Geometry check sheet. Reference: the model listing, model coordinates, mm. A direction names the side the tool comes from. Round coordinates to 2 decimals unless told otherwise and drop trailing zeros. Write each loop counter-clockwise with the first axis right and the second up, starting at its lowest first coordinate (ties: lowest second). Pieces come first, ordered by that corner, then holes. Notation, with made-up numbers: (61.25, 59.25) -> (74.25, 59.25) arc R13 cw to (74.25, 63.25) -> close; hole circle Ø4 at (-10.5, 35.5). An arc over 180 degrees is marked (long way). One line per question, with ' | ' between items.
```python
from build123d import *

# Parameters (mm, degrees)
SKETCH7_R           = 5
BOSS_EXTRUDE5_DEPTH = 12
SKETCH8_R           = 6
BOSS_EXTRUDE6_DEPTH = 2
SKETCH9_R           = 4.5
BOSS_EXTRUDE7_DEPTH = 10
FILLET2_R           = 20
FILLET3_R           = 10
FILLET5_R           = 3


with BuildPart() as part:
    # Sketch7 → Boss-Extrude5 (new body)
    with BuildSketch(Plane(origin=(0, 0, 0), x_dir=(1, 0, 0), z_dir=(0, 1, 0))):
        with BuildLine():
            Line((-105.5, 30), (-105.5, 0))
            ThreePointArc((-105.5, 0), (-95.5, -10), (-85.5, 0))
            Line((-85.5, 0), (-85.5, 15))
            Line((-85.5, 15), (-10, 15))
            Line((-10, 15), (-10, 0))
            ThreePointArc((-10, 0), (0, -10), (10, 0))
            Line((10, 0), (10, 30))
            Line((10, 30), (-10, 30))
            Line((-10, 30), (-85.5, 30))
            Line((-85.5, 30), (-105.5, 30))
        make_face()
        with Locations((-95.5, 0)):
            Circle(SKETCH7_R, mode=Mode.SUBTRACT)
    extrude(amount=BOSS_EXTRUDE5_DEPTH)

    # Sketch8 → Boss-Extrude6 (add)
    with BuildSketch(Plane(origin=(0, 12, 0), x_dir=(1, 0, 0), z_dir=(0, 1, 0))):
        Circle(SKETCH8_R)
    extrude(amount=BOSS_EXTRUDE6_DEPTH)

    # Sketch9 → Boss-Extrude7 (add)
    with BuildSketch(Plane(origin=(0, 14, 0), x_dir=(1, 0, 0), z_dir=(0, 1, 0))):
        Circle(SKETCH9_R)
    extrude(amount=BOSS_EXTRUDE7_DEPTH)

    # Fillet2
    fillet2_edges = [part.edges().sort_by_distance(p)[0] for p in [
        (-105.5, 6, -30),
        (10, 6, -30),
    ]]
    fillet(fillet2_edges, radius=FILLET2_R)

    # Fillet3
    fillet3_edges = [part.edges().sort_by_distance(p)[0] for p in [
        (-10, 6, -15),
        (-85.5, 6, -15),
    ]]
    fillet(fillet3_edges, radius=FILLET3_R)

    # Fillet5
    fillet5_edges = [part.edges().sort_by_distance(p)[0] for p in [
        (10, 0, -5),
        (-105.5, 12, -5),
        (0, 0, 10),
        (-10, 0, -2.5),
        (-85.5, 0, -2.5),
        (-95.5, 0, 10),
        (-105.5, 0, -5),
        (-95.5, 12, 10),
        (-85.5, 12, -2.5),
        (-10, 12, -2.5),
        (0, 12, 10),
        (-47.75, 0, -30),
        (-47.75, 12, -30),
        (-99.642135624, 0, -24.142135624),
        (10, 12, -5),
        (4.142135624, 0, -24.142135624),
        (-99.642135624, 12, -24.142135624),
        (4.142135624, 12, -24.142135624),
        (-47.75, 0, -15),
        (-47.75, 12, -15),
        (-12.928932188, 0, -12.071067812),
        (-12.928932188, 12, -12.071067812),
        (-82.571067812, 0, -12.071067812),
        (-82.571067812, 12, -12.071067812),
    ]]
    fillet(fillet5_edges, radius=FILLET5_R)


solid = part.part
```
(1) Sectioned sample at B-B on x = -39. Record the cut outline in (y, z).
Resolved:
outline: (0, -27) arc R3 ccw to (3, -30) -> (9, -30) arc R3 ccw to (12, -27) -> (12, -18) arc R3 ccw to (9, -15) -> (3, -15) arc R3 ccw to (0, -18) -> close
(2) Sectioned sample at D-D on y = 20.5. Record the cut outline in (x, z), then the cut area to 3 significant figures.
Resolved:
outline: circle Ø9 at (0, 0) | area: 63.6 mm2
(3) Go/stop test with flat-tipped pins: pin 1 (3 mm diameter, centred on x = -1.5, z = -19, fed in from +Y); pin 2 (5 mm diameter, centred on x = -7.5, y = 11.5, fed in from -Z); pin 3 (2 mm diameter, centred on y = 9.5, z = -24, fed in from +X); pin 4 (13 mm diameter, centred on x = -95.5, z = 0, fed in from -Y). Record where each tip stops, or that it passes through.
Resolved:
pin 1: stops at y = 12 | pin 2: stops at z = -29.94 | pin 3: stops at x = 5.16 | pin 4: stops at y = 0
(4) Material ranges on line 1 (X direction, y = 3.75, z = 0); line 2 (X direction, y = 2.75, z = -2); line 3 (Y direction, x = -89.5, z = 2.5), recorded low to high.
Resolved:
line 1: x = -105.5 to -100.5, -90.5 to -85.5, -10 to 10 | line 2: x = -105.49 to -100.08, -90.92 to -85.51, -9.99 to 9.99 | line 3: y = 0 to 12
(5) Draft check along X on faces 4 (the cylindrical face through (9.1, 0.86, -5.07)), 5 (the flat face through (0, 24, 0)), 6 (the cylindrical face through (-90.881, 5.916, 1.915)). Enter one of: +X half, -X half, draft (parallel to the pull), parting line (faces both ways), or undercut.
Resolved:
face 4: +X half | face 5: draft | face 6: undercut
(6) Access from +Z, -Z, +X, -X, +Y, -Y to the whole of each face (thin tool, end or side, straight path). Record for faces 1 (the cylindrical face through (-6, 13, 0)), 2 (the cylindrical face through (-47.36, 0.86, -15.9)), 3 (the cylindrical face through (-86.36, 11.1, -2.54)).
Resolved:
face 1: +Y | face 2: +Z, -Y | face 3: +Z, +Y
(7) Sectioned sample at A-A on z = -2. Record the cut outline in (x, y), then the cut area to 3 significant figures.
Resolved:
outline: (-105.5, 3) arc R3 ccw to (-102.5, 0) -> (-100.08, 0) -> (-100.08, 12) -> (-102.5, 12) arc R3 ccw to (-105.5, 9) -> close; (-90.92, 0) -> (-88.5, 0) arc R3 ccw to (-85.5, 3) -> (-85.5, 9) arc R3 ccw to (-88.5, 12) -> (-90.92, 12) -> close; (-10, 3) arc R3 ccw to (-7, 0) -> (7, 0) arc R3 ccw to (10, 3) -> (10, 9) arc R3 ccw to (7, 12) -> (5.66, 12) -> (5.66, 14) -> (4.03, 14) -> (4.03, 24) -> (-4.03, 24) -> (-4.03, 14) -> (-5.66, 14) -> (-5.66, 12) -> (-7, 12) arc R3 ccw to (-10, 9) -> close | area: 458 mm2
(8) Sectioned sample at C-C on y = 10.75. Record the cut outline in (x, z), then the cut area to 3 significant figures.
Resolved:
outline: (-104.94, -10) arc R19.44 ccw to (-85.5, -29.44) -> (-10, -29.44) arc R19.44 ccw to (9.44, -10) -> (9.44, 0) arc R9.44 ccw to (-9.44, 0) -> (-9.44, -5) arc R10.56 cw to (-20, -15.56) -> (-75.5, -15.56) arc R10.56 cw to (-86.06, -5) -> (-86.06, 0) arc R9.44 ccw to (-104.94, 0) -> close; hole circle Ø10 at (-95.5, 0) | area: 2,260 mm2
